Answer from the drawing. Dimensions are ordinates in mm from the lowest x, y and z of the part. A direction names the side the tool comes from. Coordinates: 2 decimals unless noted, no trailing zeros. Write each loop counter-clockwise with the first axis right and the second up, starting at its lowest first coordinate (ties: lowest second). Pieces come first, ordered by that corner, then holes.
1) The part is cut by section C-C (x = 25). Determine the outline of the cut face in (y, z).
2) The part is cut by section B-B (z = 2.1). Determine the outline of the cut face in (x, y), then the cut area to 3 significant figures.
3) The part is cut by section D-D (y = 9.5). Determine the outline of the cut face in (x, z).
4) The part is cut by section A-A (y = 18.9). Determine the outline of the cut face in (x, z).
5) Determine the mould class of the marked faces 3, 4 and 5 for opening direction Y: +Y half, -Y half, draft (parallel to the pull), parting line (faces both ways), or undercut.
6) Find the intervals of material crossed by line 1 (Y direction, x = 17.5, z = 3.6); line 2 (X direction, y = 18.75, z = 2); line 3 (Y direction, x = 13.6, z = 1.3), in increasing order.
7) Which of the six approach directions +Z, -Z, +X, -X, +Y, -Y give full straight-line access (tool end or side, diameter ignored) to the marked faces 1 and 2?
8) This flat-tipped pin is pushed along its axis until it touches: pin 1 Ø1.2 at (x, y) = (13.6, 6.1) entering from +Z. Where does it stop, or does it pass through?
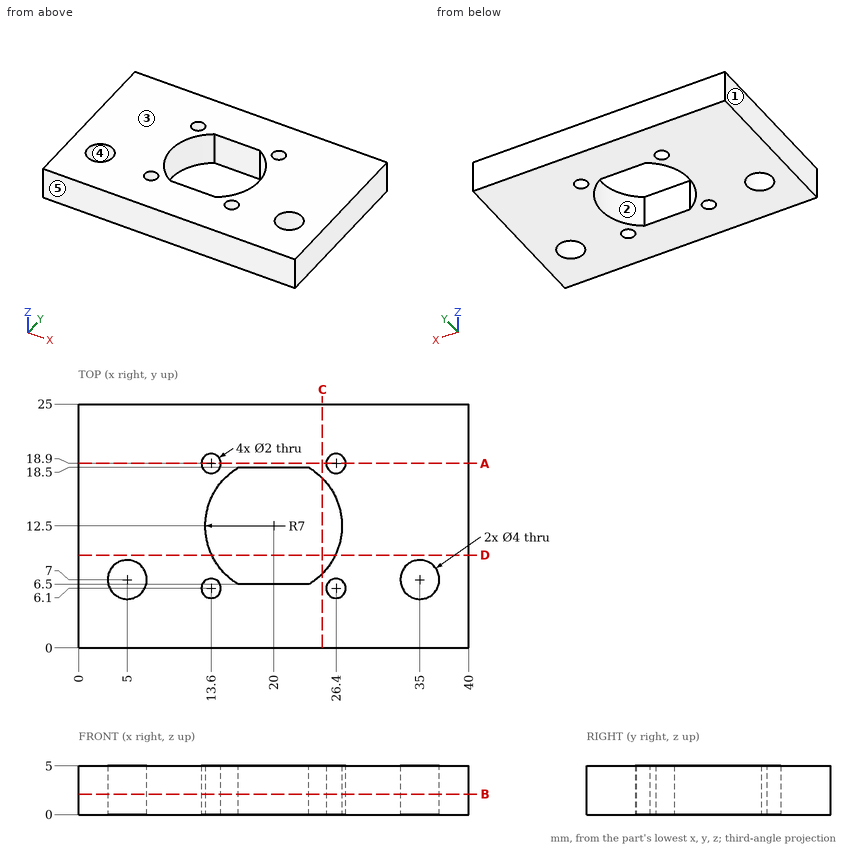
Reported:
1. outline: (0, 0) - (7.6, 0) - (7.6, 5) - (0, 5) - close; (17.4, 0) - (25, 0) - (25, 5) - (17.4, 5) - close
2. outline: (0, 0) - (40, 0) - (40, 25) - (0, 25) - close; hole circle Ø4 at (5, 7); hole circle Ø2 at (13.6, 6.1); hole circle Ø2 at (13.6, 18.9); hole (16.39, 6.5) - (23.61, 6.5) arc R7 ccw to (23.61, 18.5) - (16.39, 18.5) arc R7 ccw to start; hole circle Ø2 at (26.4, 6.1); hole circle Ø2 at (26.4, 18.9); hole circle Ø4 at (35, 7)
2. area: 818 mm2
3. outline: (0, 0) - (13.68, 0) - (13.68, 5) - (0, 5) - close; (26.32, 0) - (40, 0) - (40, 5) - (26.32, 5) - close
4. outline: (0, 0) - (12.6, 0) - (12.6, 5) - (0, 5) - close; (14.6, 0) - (25.4, 0) - (25.4, 5) - (14.6, 5) - close; (27.4, 0) - (40, 0) - (40, 5) - (27.4, 5) - close
5. face 3: draft
5. face 4: undercut
5. face 5: -Y half
6. line 1: y = 0 to 6.5, 18.5 to 25
6. line 2: x = 0 to 12.61, 14.59 to 25.41, 27.39 to 40
6. line 3: y = 0 to 5.1, 7.1 to 9.66, 15.34 to 17.9, 19.9 to 25
7. face 1: +Z, -Z, -X, +Y, -Y
7. face 2: +Z, -Z
8. pin 1: passes through
